```python
from build123d import *

# Parameters (mm, degrees)
SKETCH1_W             = 114.3
SKETCH1_H             = 203.2
BOSS_EXTRUDE1_DEPTH   = 33.02
SKETCH2_W             = 26.67
SKETCH2_H             = 25.4
CUT_EXTRUDE1_DEPTH    = 204.2
CHAMFER1_SIZE         = 17.62
CHAMFER1_SIZE2        = 26.122724265
CHAMFER1_PART_2_SIZE  = 17.62
CHAMFER1_PART_2_SIZE2 = 26.122724265
SKETCH3_W             = 5.08
SKETCH3_H             = 203.2
BOSS_EXTRUDE2_DEPTH   = 20.32
CHAMFER2_SIZE         = 17.62
CHAMFER2_SIZE2        = 26.122724265
CHAMFER2_PART_2_SIZE  = 17.62
CHAMFER2_PART_2_SIZE2 = 26.122724265
SKETCH5_W             = 76.2
SKETCH5_H             = 76.2
CUT_EXTRUDE2_DEPTH    = 2.54


with BuildPart() as part:
    # Sketch1 → Boss-Extrude1 (new body)
    with BuildSketch(Plane.XY):
        with Locations((97.239666667, -13.292666667)):
            Rectangle(SKETCH1_W, SKETCH1_H)
    extrude(amount=BOSS_EXTRUDE1_DEPTH)

    # Sketch2 → Cut-Extrude1 (cut, through all)
    with BuildSketch(Plane(origin=(0, 88.307333333, 0), x_dir=(1, 0, 0), z_dir=(0, 1, 0))):
        with Locations((53.424666667, -20.32)):
            Rectangle(SKETCH2_W, SKETCH2_H)
        with Locations((141.054666667, -20.32)):
            Rectangle(SKETCH2_W, SKETCH2_H)
    extrude(amount=-CUT_EXTRUDE1_DEPTH, mode=Mode.SUBTRACT)

    # Chamfer1
    chamfer1_edges = [part.edges().sort_by_distance(p)[0] for p in [
        (97.239666667, -114.892666667, 33.02),
    ]]
    chamfer1_side = [part.faces().sort_by_distance(p)[0] for p in [
        (97.239666667, -114.892666667, 14.3764),
    ]]
    chamfer(chamfer1_edges, length=CHAMFER1_SIZE, length2=CHAMFER1_SIZE2, reference=chamfer1_side[0])

    # Chamfer1 part 2
    chamfer1_part_2_edges = [part.edges().sort_by_distance(p)[0] for p in [
        (97.239666667, 88.307333333, 33.02),
    ]]
    chamfer1_part_2_side = [part.faces().sort_by_distance(p)[0] for p in [
        (97.239666667, 88.307333333, 14.3764),
    ]]
    chamfer(chamfer1_part_2_edges, length=CHAMFER1_PART_2_SIZE, length2=CHAMFER1_PART_2_SIZE2, reference=chamfer1_part_2_side[0])

    # Sketch3 → Boss-Extrude2 (add)
    with BuildSketch(Plane.XY.offset(7.62)):
        with Locations((42.629666667, -13.292666667)):
            Rectangle(SKETCH3_W, SKETCH3_H)
        with Locations((151.849666667, -13.292666667)):
            Rectangle(SKETCH3_W, SKETCH3_H)
    extrude(amount=BOSS_EXTRUDE2_DEPTH)

    # Chamfer2
    chamfer2_edges = [part.edges().sort_by_distance(p)[0] for p in [
        (42.629666667, -114.892666667, 27.94),
        (151.849666667, -114.892666667, 27.94),
    ]]
    chamfer2_side = [part.faces().sort_by_distance(p)[0] for p in [
        (97.239666667, -114.892666667, 8.022187919),
    ]]
    chamfer(chamfer2_edges, length=CHAMFER2_SIZE, length2=CHAMFER2_SIZE2, reference=chamfer2_side[0])

    # Chamfer2 part 2
    chamfer2_part_2_edges = [part.edges().sort_by_distance(p)[0] for p in [
        (42.629666667, 88.307333333, 27.94),
        (151.849666667, 88.307333333, 27.94),
    ]]
    chamfer2_part_2_side = [part.faces().sort_by_distance(p)[0] for p in [
        (97.239666667, 88.307333333, 8.022187919),
    ]]
    chamfer(chamfer2_part_2_edges, length=CHAMFER2_PART_2_SIZE, length2=CHAMFER2_PART_2_SIZE2, reference=chamfer2_part_2_side[0])

    # Sketch5 → Cut-Extrude2 (cut)
    with BuildSketch(Plane(origin=(0, 0, 0), x_dir=(-1, 0, 0), z_dir=(0, 0, -1))):
        with Locations((-97.239666667, 24.807333333)):
            Rectangle(SKETCH5_W, SKETCH5_H)
    extrude(amount=-CUT_EXTRUDE2_DEPTH, mode=Mode.SUBTRACT)


solid = part.part
```
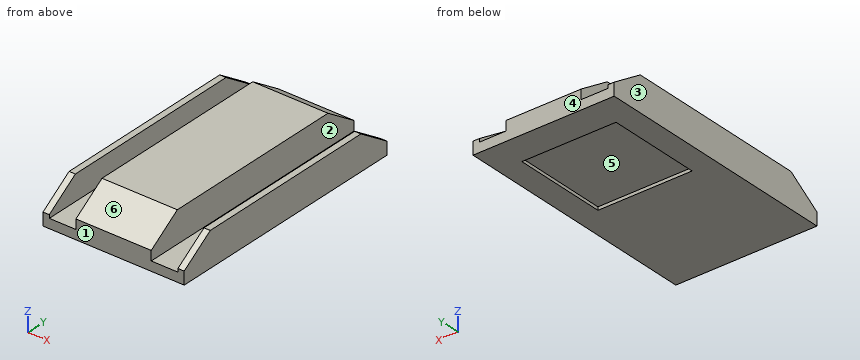
Input: part model. Units: mm. Frame: model coordinates. Face numbers are marked on the shaded views. A direction names the side the tool comes from. Coordinates: 2 decimals unless noted, no trailing zeros. Write each loop counter-clockwise with the first axis right and the second up, starting at its lowest first coordinate (ties: lowest second). Pieces come first, ordered by that corner, then holes.
1) Pin query (flat end, axial travel): pin 1 Ø4 at (x, z) = (112, 25) entering from -Y; pin 2 Ø2.5 at (x, y) = (41.5, -50) entering from +Z; pin 3 Ø1.5 at (x, z) = (123.5, 29.5) entering from +Y. Return the tip coordinate at first contact, or that it passes through.
2) Material intervals for line 1 along X through (y, z) = (-17.5, 14); line 2 along Y through (x, z) = (72, 2.5); line 3 along Z through (x, y) = (53, 67.5), sorted ascending.
3) Section C-C on y = -67. Output: boundary loops of the cut face in (x, z).
4) Section D-D on y = 72.5. Output: boundary loops of the cut face in (x, z), and give its area (3 significant figures).
5) Mould query, pull axis Y, two halves, no side actions, for the marked faces 3, 4, 5 and 6. Classes: pulls with the +Y half, pulls with the -Y half, needs draft (parallel to the pull), parting line crosses it, or undercut.
6) Section A-A on y = 48. Output: boundary loops of the cut face in (x, z).
7) Set-up query: the marked faces 1 and 2. Return all of +Z, -Z, +X, -X, +Y, -Y with unobstructed straight access to the full face (end or side cutting, diameter ignored); none if empty.
8) Section B-B on x = 110. Output: boundary loops of the cut face in (y, z), and give its area (3 significant figures).
Check result:
1. pin 1: stops at y = -103.63
1. pin 2: stops at z = 27.94
1. pin 3: stops at y = 68.52
2. line 1: x = 40.09 to 45.17, 66.76 to 127.72, 149.31 to 154.39
2. line 2: y = -114.89 to -13.29, 62.91 to 88.31
2. line 3: z = 0 to 7.62
3. outline: (40.09, 0) - (154.39, 0) - (154.39, 27.94) - (149.31, 27.94) - (149.31, 7.62) - (127.72, 7.62) - (127.72, 33.02) - (66.76, 33.02) - (66.76, 7.62) - (45.17, 7.62) - (45.17, 27.94) - (40.09, 27.94) - close
4. outline: (40.09, 0) - (154.39, 0) - (154.39, 20.98) - (149.31, 20.98) - (149.31, 7.62) - (127.72, 7.62) - (127.72, 26.06) - (66.76, 26.06) - (66.76, 7.62) - (45.17, 7.62) - (45.17, 20.98) - (40.09, 20.98) - close
4. area: 2,130 mm2
5. face 3: needs draft
5. face 4: pulls with the +Y half
5. face 5: undercut
5. face 6: pulls with the -Y half
6. outline: (40.09, 0) - (59.14, 0) - (59.14, 2.54) - (135.34, 2.54) - (135.34, 0) - (154.39, 0) - (154.39, 27.94) - (149.31, 27.94) - (149.31, 7.62) - (127.72, 7.62) - (127.72, 33.02) - (66.76, 33.02) - (66.76, 7.62) - (45.17, 7.62) - (45.17, 27.94) - (40.09, 27.94) - close
7. face 1: +Z, -Z, +X, -X, -Y
7. face 2: +Z, +Y, -Y
8. outline: (-114.89, 0) - (-13.29, 0) - (-13.29, 2.54) - (62.91, 2.54) - (62.91, 0) - (88.31, 0) - (88.31, 15.4) - (62.18, 33.02) - (-88.77, 33.02) - (-114.89, 15.4) - close
8. area: 6,060 mm2
